Could you check a few things on this model? Use its own coordinates, in mm. A direction names the side the tool comes from. Coordinates: 2 decimals unless noted, no trailing zeros. Loops run counter-clockwise (first coordinate to the right, second up) from the corner with the lowest first, then second, coordinate; pieces in that order, holes last.
Autodesk Inventor part; units mm, degrees
ref_plane "Work Plane1" through (0, 2, 0) normal (0, -1, 0) x (1, 0, 0)
ref_plane "YZ Plane" through (0, 0, 0) normal (1, 0, 0) x (0, 1, 0)
ref_plane "XZ Plane" through (0, 0, 0) normal (0, 1, 0) x (-1, 0, 0)
sketch "Sketch1" plane through (0, 0, 0) normal (0, 1, 0) x (-1, 0, 0)
  line L0 (-4.3, 2.15) -> (4.3, 2.15)
  line L1 (4.3, 2.15) -> (4.3, -2.15)
  line L2 (4.3, -2.15) -> (-4.3, -2.15)
  line L3 (-4.3, -2.15) -> (-4.3, 2.15)
  line L4 (-4.3, 2.15) -> (4.3, -2.15) construction
  line L5 (4.3, 2.15) -> (-4.3, -2.15) construction
  point P0 (0, 0)
  dimension "d0" = 8.6
  dimension "d1" = 4.3
extrude "Extrusion1" add sketch "Sketch1" along normal blind 3.5
sketch "Sketch2" plane through (0, 0, 0) normal (0, -1, 0) x (1, 0, 0)
  circle A0 centre (0, 0) radius 0.4
  circle A1 centre (2, 0) radius 0.4
  circle A2 centre (-2, 0) radius 0.4
  circle A3 centre (-4, 0) radius 0.5
  circle A4 centre (4, 0) radius 0.5
  dimension "d4" = 0.8
  dimension "d5" = 0.8
  dimension "d6" = 0.8
  dimension "d7" = 2
  dimension "d8" = 2
  dimension "d9" = 1
  dimension "d10" = 1
  dimension "d11" = 2
  dimension "d12" = 2
extrude "Extrusion2" add sketch "Sketch2" along normal blind 2.77
ref_plane "Work Plane1" through (0, 2, 0) normal (0, -1, 0) x (1, 0, 0)
sketch "Sketch3" plane through (0, 2, 0) normal (0, -1, 0) x (1, 0, 0)
  line L0 (-2, -2.15) -> (-2, -5.15)
  line L1 (-2, -5.15) -> (0, -5.15)
  line L2 (-2, -2.15) -> (0, -2.15)
  line L3 (0, -2.15) -> (0, -5.15)
  line L4 (-4.3, -2.15) -> (4.3, -2.15)
  point P0 (0, 0)
  dimension "d16" = 2
  dimension "d17" = 0
  dimension "d18" = 0
  dimension "d19" = 3
extrude "Extrusion3" add sketch "Sketch3" along normal mid plane 2
properties part number "TE-1825232"
(1) Which directions (+Z, -Z, +X, -X, +Y, -Y) give clear straight access to the entire face, cutting with the end or side of a thin tool? Please do faces 4 (the face through (0, 0, 1)), 5 (the face through (-2, 2, -4)), 6 (the face through (-1, 1, -4)), 7 (the face through (-1, 3, -4)), 8 (the face through (0, 2, -4)).
Answers:
face 4: -Y
face 5: -Z, -X, +Y, -Y
face 6: -Z, +X, -X, -Y
face 7: -Z, +X, -X, +Y
face 8: -Z, +X, +Y, -Y
(2) We'd pull the mould along X, two halves only. Please class faces 1 (the face through (-4.4, -1.4, 0.3)), 2 (the face through (-4.3, 2, 0)), 3 (the face through (1, 2, -2.15)): +X half, -X half, draft (parallel to the pull), parting line (faces both ways), or undercut.
Answers:
face 1: undercut
face 2: -X half
face 3: draft
(3) I need wall thicknesses on probe 1 along X at (y, z) = (2, -2); probe 2 along Y at (x, z) = (-1, 0); probe 3 along Z at (x, y) = (1.25, 1). Which ranges of each line are inside material? Lowest first, please.
Answers:
probe 1: x = -4.3 to 4.3
probe 2: y = 0 to 3.5
probe 3: z = -2.15 to 2.15
(4) Imagine slicing it at D-D, the plane x = -3. Write out the boundary of the cut face in (y, z), and give its area (4 significant figures).
Answers:
outline: (0, -2.15) - (3.5, -2.15) - (3.5, 2.15) - (0, 2.15) - close
area: 15.05 mm2
(5) Imagine slicing it at A-A, the plane y = 2.75. Write out the boundary of the cut face in (x, z).
Answers:
outline: (-4.3, -2.15) - (-2, -2.15) - (-2, -5.15) - (0, -5.15) - (0, -2.15) - (4.3, -2.15) - (4.3, 2.15) - (-4.3, 2.15) - close
(6) Imagine slicing it at B-B, the plane z = 0. Write out the boundary of the cut face in (x, y).
Answers:
outline: (-4.5, -2.77) - (-3.5, -2.77) - (-3.5, 0) - (-2.4, 0) - (-2.4, -2.77) - (-1.6, -2.77) - (-1.6, 0) - (-0.4, 0) - (-0.4, -2.77) - (0.4, -2.77) - (0.4, 0) - (1.6, 0) - (1.6, -2.77) - (2.4, -2.77) - (2.4, 0) - (3.5, 0) - (3.5, -2.77) - (4.5, -2.77) - (4.5, 0) - (4.3, 0) - (4.3, 3.5) - (-4.3, 3.5) - (-4.3, 0) - (-4.5, 0) - close
(7) For pin 1 (1 mm diameter, centred on y = 1.5, z = 1, fed in from +X); pin 2 (1 mm diameter, centred on x = -1.5, z = -3, fed in from +Y); pin 3 (1 mm diameter, centred on y = 2.5, z = 0, fed in from -X); pin 4 (1 mm diameter, centred on x = -3.5, z = -3, fed in from +Y), each with a flat end and sliding along its axis, tell me the tip position at first contact or that it passes through.
Answers:
pin 1: stops at x = 4.3
pin 2: stops at y = 3
pin 3: stops at x = -4.3
pin 4: passes through
(8) Imagine slicing it at C-C, the plane x = 0.25. Write out the boundary of the cut face in (y, z), and give its area (3 significant figures).
Answers:
outline: (-2.77, -0.31) - (0, -0.31) - (0, -2.15) - (3.5, -2.15) - (3.5, 2.15) - (0, 2.15) - (0, 0.31) - (-2.77, 0.31) - close
area: 16.8 mm2
